Autodesk Inventor part; units mm, degrees
ref_plane "YZ Plane" through (0, 0, 0) normal (1, 0, 0) x (0, 1, 0)
ref_plane "XZ Plane" through (0, 0, 0) normal (0, 1, 0) x (-1, 0, 0)
ref_plane "XY Plane" through (0, 0, 0) normal (0, 0, 1) x (1, 0, 0)
sketch "Sketch3" plane through (0, 0, 0) normal (0, 0, 1) x (1, 0, 0)
  circle A0 centre (0, 0) radius 1.5
  dimension "Diameter" = 3
extrude "Extrusion1" add sketch "Sketch3" against normal blind 25
sketch "Sketch4" plane through (0, 0, 0) normal (0, 0, 1) x (1, 0, 0)
  circle A0 centre (0, 0) radius 1.5
  circle A1 centre (0, 0) radius 2.75
  dimension "Head_Diameter" = 5.5
extrude "Extrusion2" add sketch "Sketch4" along normal blind 3 contours A0 | A1
sketch "Sketch5" plane through (0, 0, 3) normal (0, 0, 1) x (1, 0, 0)
  circle A0 centre (0, 0) radius 2.75
  line L0 (1.4434, 0) -> (0.7217, -1.25)
  line L1 (0.7217, -1.25) -> (-0.7217, -1.25)
  line L2 (-0.7217, -1.25) -> (-1.4434, 0)
  line L3 (-1.4434, 0) -> (-0.7217, 1.25)
  line L4 (-0.7217, 1.25) -> (0.7217, 1.25)
  line L5 (0.7217, 1.25) -> (1.4434, 0)
  line L6 (0, 0) -> (1.4434, 0) construction
  dimension "Hex_Width" = 2.5
extrude "Extrusion3" cut sketch "Sketch5" against normal blind 1.5 contours L0 L1 L2 L3 L4 L5
thread "Thread1"
chamfer "Chamfer1" distance 0.3 angle 45 1 edges at (-2.75, 0, 3)
chamfer "Chamfer2" distance 0.15 angle 45 1 edges at (-1.5, 0, -25)
equation "\"d14\" = 0.5 * Chamfer"
properties part number "SCREW,SOCKET-HD,P,12_9,M03X0_5X25MM" material "Steel, MS"
Check sheet for the modelled part. Datum: model origin and axes. Units: mm. A direction names the side the tool comes from. Give positions to 0.01 mm unless a question says otherwise; leave off trailing zeros. Write each loop counter-clockwise with the first axis right and the second up, starting at its lowest first coordinate (ties: lowest second). Pieces come first, ordered by that corner, then holes. Notation, with made-up numbers: (19, 17) - (75, 17) arc R14 cw to (75, 33) - close; hole circle Ø4 at (89, 50.5). An arc over 180 degrees is marked (long way). Answer as a JSON object with one key per item and string values. Group by question number.
1) Sectioned sample at A-A (x = 0). Record the cut outline in (y, z).
2) Access from +Z, -Z, +X, -X, +Y, -Y to the whole of each face (thin tool, end or side, straight path). Record for faces 1 (the face through (0, -1.25, 2)), 2 (the face through (-1.5, 0.07, -12.25)), 3 (the face through (0, 0, -25)).
3) Release check for a two-part mould opening along X. For faces 4 (the face through (1.08, 0.63, 2.26)), 5 (the face through (1.2, -1.2, 0)), 6 (the face through (-0.596, 2.685, 1.331)) record: pulls with the +X half, pulls with the -X half, needs draft (parallel to the pull), parting line crosses it, or undercut.
4) Thickness scan on probe 1 along Z at (x, y) = (0.9, 0); probe 2 along Y at (x, z) = (0.65, -7); probe 3 along Z at (x, y) = (-1.7, -1). Record the ranges inside material, lowest first. Write a range as from..to.
5) Sectioned sample at B-B (z = -5.25). Record the cut outline in (x, y), then the cut area to 3 significant figures.
Geometry results:
{
 "1": {"outline": "(-2.75, 0) - (-1.5, 0) - (-1.5, -24.85) - (-1.35, -25) - (1.35, -25) - (1.5, -24.85) - (1.5, 0) - (2.75, 0) - (2.75, 2.7) - (2.45, 3) - (1.25, 3) - (1.25, 1.5) - (-1.25, 1.5) - (-1.25, 3) - (-2.45, 3) - (-2.75, 2.7) - close"},
 "2": {"face 1": "+Z", "face 2": "-Z", "face 3": "-Z, +X, -X, +Y, -Y"},
 "3": {"face 4": "undercut", "face 5": "needs draft", "face 6": "parting line crosses it"},
 "4": {"probe 1": "z = -25..1.5", "probe 2": "y = -1.35..1.35", "probe 3": "z = 0..3"},
 "5": {"outline": "circle Ø3 at (0, 0)", "area": "7.07 mm^2"}
}
